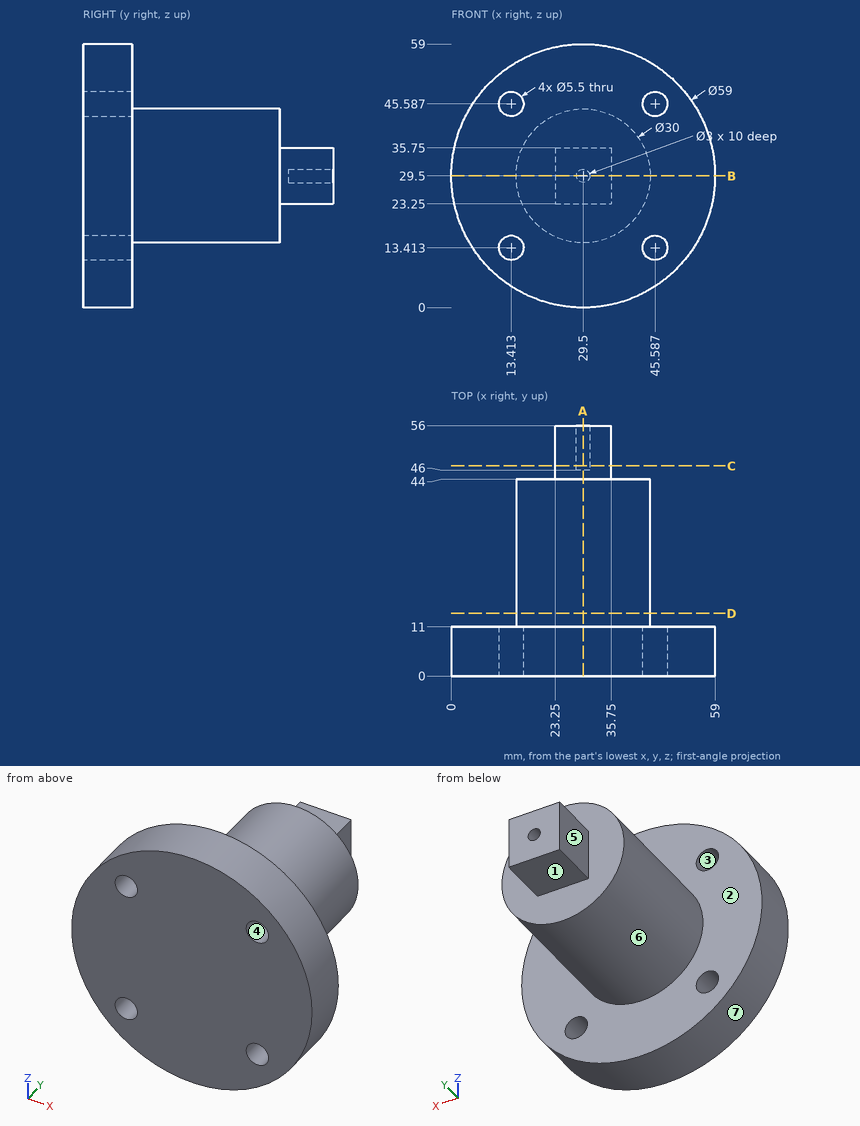
Print and shaded views of the part. All mm, measured from the part's lowest x, y and z. A direction names the side the tool comes from. Coordinates: 2 decimals unless noted, no trailing zeros. Order: outer loops, then holes, each group sorted by start corner. A loop starts at its lowest first (then second) coordinate and runs counter-clockwise, first axis right, second up.
(1) Slice it at B-B, the plane z = 29.5. Write the cut outline in (x, y).
Check sheet entries:
outline: (0, 0) - (59, 0) - (59, 11) - (44.5, 11) - (44.5, 44) - (35.75, 44) - (35.75, 56) - (31, 56) - (31, 46) - (28, 46) - (28, 56) - (23.25, 56) - (23.25, 44) - (14.5, 44) - (14.5, 11) - (0, 11) - close
(2) Probe L1, parallel to X at y = 52, z = 29.5; L2, parallel to Z at x = 12.5, y = 5. List the from-to ranges inside material, lowest first.
Check sheet entries:
L1: x = 23.25 to 28, 31 to 35.75
L2: z = 5.39 to 10.82, 16.01 to 42.99, 48.18 to 53.61
(3) Slice it at D-D, the plane y = 14. Write the cut outline in (x, z).
Check sheet entries:
outline: circle Ø30 at (29.5, 29.5)
(4) Slice it at C-C, the plane y = 47. Write the cut outline in (x, z).
Check sheet entries:
outline: (23.25, 23.25) - (35.75, 23.25) - (35.75, 35.75) - (23.25, 35.75) - close; hole circle Ø3 at (29.5, 29.5)
(5) Slice it at A-A, the plane x = 29.5. Write the cut outline in (y, z).
Check sheet entries:
outline: (0, 0) - (11, 0) - (11, 14.5) - (44, 14.5) - (44, 23.25) - (56, 23.25) - (56, 28) - (46, 28) - (46, 31) - (56, 31) - (56, 35.75) - (44, 35.75) - (44, 44.5) - (11, 44.5) - (11, 59) - (0, 59) - close
(6) Pin check, flat tips, straight feed: pin 1 Ø2 at (y, z) = (39.5, 37.5) entering from +X; pin 2 Ø13 at (y, z) = (53, 31.5) entering from +X; pin 3 Ø6 at (x, y) = (32.5, 51.5) entering from +Z. Stop position of each tip, or through.
Check sheet entries:
pin 1: stops at x = 42.77
pin 2: stops at x = 35.75
pin 3: stops at z = 35.75
(7) Pull direction Z, two halves, no side cores. Call the marked faces 1, 2, 3 and 4: pulls with the +Z half, pulls with the -Z half, needs draft (parallel to the pull), parting line crosses it, or undercut.
Check sheet entries:
face 1: pulls with the -Z half
face 2: needs draft
face 3: undercut
face 4: undercut
(8) Tool access for the marked faces 5, 6 and 7: list every direction of +Z, -Z, +X, -X, +Y, -Y with a clear straight run to the whole face (end or side of a thin tool).
Check sheet entries:
face 5: +Z, -Z, -X, +Y
face 6: +Y
face 7: +Y, -Y
